```python
from build123d import *

# Parameters (mm, degrees)
SKETCH_1_W      = 100
SKETCH_1_H      = 70
EXTRUDE_1_DEPTH = 3.2


with BuildPart() as part:
    # Эскиз1 → Бобышка-Вытянуть1 (new body)
    with BuildSketch(Plane(origin=(0, 0, 0), x_dir=(1, 0, 0), z_dir=(0, 1, 0))):
        Rectangle(SKETCH_1_W, SKETCH_1_H)
        with BuildLine():
            Line((-42.453867058, 30.513030215), (-33.354611201, 5.513030215))
            ThreePointArc((-33.354611201, 5.513030215), (-34.251119917, 3.590461069), (-36.173689063, 4.486969785))
            Line((-36.173689063, 4.486969785), (-45.27294492, 29.486969785))
            ThreePointArc((-45.27294492, 29.486969785), (-44.376436204, 31.409538931), (-42.453867058, 30.513030215))
        make_face(mode=Mode.SUBTRACT)
        with BuildLine():
            Line((-32.453867058, 30.513030215), (-23.354611201, 5.513030215))
            ThreePointArc((-23.354611201, 5.513030215), (-24.251119917, 3.590461069), (-26.173689063, 4.486969785))
            Line((-26.173689063, 4.486969785), (-35.27294492, 29.486969785))
            ThreePointArc((-35.27294492, 29.486969785), (-34.376436204, 31.409538931), (-32.453867058, 30.513030215))
        make_face(mode=Mode.SUBTRACT)
        with BuildLine():
            Line((-22.453867058, 30.513030215), (-13.354611201, 5.513030215))
            ThreePointArc((-13.354611201, 5.513030215), (-14.251119917, 3.590461069), (-16.173689063, 4.486969785))
            Line((-16.173689063, 4.486969785), (-25.27294492, 29.486969785))
            ThreePointArc((-25.27294492, 29.486969785), (-24.376436204, 31.409538931), (-22.453867058, 30.513030215))
        make_face(mode=Mode.SUBTRACT)
        with BuildLine():
            Line((-12.453867058, 30.513030215), (-3.354611201, 5.513030215))
            ThreePointArc((-3.354611201, 5.513030215), (-4.251119917, 3.590461069), (-6.173689063, 4.486969785))
            Line((-6.173689063, 4.486969785), (-15.27294492, 29.486969785))
            ThreePointArc((-15.27294492, 29.486969785), (-14.376436204, 31.409538931), (-12.453867058, 30.513030215))
        make_face(mode=Mode.SUBTRACT)
        with BuildLine():
            Line((-2.453867058, 30.513030215), (6.645388799, 5.513030215))
            ThreePointArc((6.645388799, 5.513030215), (5.748880083, 3.590461069), (3.826310937, 4.486969785))
            Line((3.826310937, 4.486969785), (-5.27294492, 29.486969785))
            ThreePointArc((-5.27294492, 29.486969785), (-4.376436204, 31.409538931), (-2.453867058, 30.513030215))
        make_face(mode=Mode.SUBTRACT)
        with BuildLine():
            Line((7.546132942, 30.513030215), (16.645388799, 5.513030215))
            ThreePointArc((16.645388799, 5.513030215), (15.748880083, 3.590461069), (13.826310937, 4.486969785))
            Line((13.826310937, 4.486969785), (4.72705508, 29.486969785))
            ThreePointArc((4.72705508, 29.486969785), (5.623563796, 31.409538931), (7.546132942, 30.513030215))
        make_face(mode=Mode.SUBTRACT)
        with BuildLine():
            Line((17.546132942, 30.513030215), (26.645388799, 5.513030215))
            ThreePointArc((26.645388799, 5.513030215), (25.748880083, 3.590461069), (23.826310937, 4.486969785))
            Line((23.826310937, 4.486969785), (14.72705508, 29.486969785))
            ThreePointArc((14.72705508, 29.486969785), (15.623563796, 31.409538931), (17.546132942, 30.513030215))
        make_face(mode=Mode.SUBTRACT)
        with BuildLine():
            Line((27.546132942, 30.513030215), (36.645388799, 5.513030215))
            ThreePointArc((36.645388799, 5.513030215), (35.748880083, 3.590461069), (33.826310937, 4.486969785))
            Line((33.826310937, 4.486969785), (24.72705508, 29.486969785))
            ThreePointArc((24.72705508, 29.486969785), (25.623563796, 31.409538931), (27.546132942, 30.513030215))
        make_face(mode=Mode.SUBTRACT)
        with BuildLine():
            Line((37.546132942, 30.513030215), (46.645388799, 5.513030215))
            ThreePointArc((46.645388799, 5.513030215), (45.748880083, 3.590461069), (43.826310937, 4.486969785))
            Line((43.826310937, 4.486969785), (34.72705508, 29.486969785))
            ThreePointArc((34.72705508, 29.486969785), (35.623563796, 31.409538931), (37.546132942, 30.513030215))
        make_face(mode=Mode.SUBTRACT)
        with BuildLine():
            Line((-2.453867058, -30.513030215), (6.645388799, -5.513030215))
            ThreePointArc((6.645388799, -5.513030215), (5.748880083, -3.590461069), (3.826310937, -4.486969785))
            Line((3.826310937, -4.486969785), (-5.27294492, -29.486969785))
            ThreePointArc((-5.27294492, -29.486969785), (-4.376436204, -31.409538931), (-2.453867058, -30.513030215))
        make_face(mode=Mode.SUBTRACT)
        with BuildLine():
            Line((37.546132942, -30.513030215), (46.645388799, -5.513030215))
            ThreePointArc((46.645388799, -5.513030215), (45.748880083, -3.590461069), (43.826310937, -4.486969785))
            Line((43.826310937, -4.486969785), (34.72705508, -29.486969785))
            ThreePointArc((34.72705508, -29.486969785), (35.623563796, -31.409538931), (37.546132942, -30.513030215))
        make_face(mode=Mode.SUBTRACT)
        with BuildLine():
            Line((27.546132942, -30.513030215), (36.645388799, -5.513030215))
            ThreePointArc((36.645388799, -5.513030215), (35.748880083, -3.590461069), (33.826310937, -4.486969785))
            Line((33.826310937, -4.486969785), (24.72705508, -29.486969785))
            ThreePointArc((24.72705508, -29.486969785), (25.623563796, -31.409538931), (27.546132942, -30.513030215))
        make_face(mode=Mode.SUBTRACT)
        with BuildLine():
            Line((17.546132942, -30.513030215), (26.645388799, -5.513030215))
            ThreePointArc((26.645388799, -5.513030215), (25.748880083, -3.590461069), (23.826310937, -4.486969785))
            Line((23.826310937, -4.486969785), (14.72705508, -29.486969785))
            ThreePointArc((14.72705508, -29.486969785), (15.623563796, -31.409538931), (17.546132942, -30.513030215))
        make_face(mode=Mode.SUBTRACT)
        with BuildLine():
            Line((7.546132942, -30.513030215), (16.645388799, -5.513030215))
            ThreePointArc((16.645388799, -5.513030215), (15.748880083, -3.590461069), (13.826310937, -4.486969785))
            Line((13.826310937, -4.486969785), (4.72705508, -29.486969785))
            ThreePointArc((4.72705508, -29.486969785), (5.623563796, -31.409538931), (7.546132942, -30.513030215))
        make_face(mode=Mode.SUBTRACT)
        with BuildLine():
            Line((-12.453867058, -30.513030215), (-3.354611201, -5.513030215))
            ThreePointArc((-3.354611201, -5.513030215), (-4.251119917, -3.590461069), (-6.173689063, -4.486969785))
            Line((-6.173689063, -4.486969785), (-15.27294492, -29.486969785))
            ThreePointArc((-15.27294492, -29.486969785), (-14.376436204, -31.409538931), (-12.453867058, -30.513030215))
        make_face(mode=Mode.SUBTRACT)
        with BuildLine():
            Line((-22.453867058, -30.513030215), (-13.354611201, -5.513030215))
            ThreePointArc((-13.354611201, -5.513030215), (-14.251119917, -3.590461069), (-16.173689063, -4.486969785))
            Line((-16.173689063, -4.486969785), (-25.27294492, -29.486969785))
            ThreePointArc((-25.27294492, -29.486969785), (-24.376436204, -31.409538931), (-22.453867058, -30.513030215))
        make_face(mode=Mode.SUBTRACT)
        with BuildLine():
            Line((-32.453867058, -30.513030215), (-23.354611201, -5.513030215))
            ThreePointArc((-23.354611201, -5.513030215), (-24.251119917, -3.590461069), (-26.173689063, -4.486969785))
            Line((-26.173689063, -4.486969785), (-35.27294492, -29.486969785))
            ThreePointArc((-35.27294492, -29.486969785), (-34.376436204, -31.409538931), (-32.453867058, -30.513030215))
        make_face(mode=Mode.SUBTRACT)
        with BuildLine():
            Line((-42.453867058, -30.513030215), (-33.354611201, -5.513030215))
            ThreePointArc((-33.354611201, -5.513030215), (-34.251119917, -3.590461069), (-36.173689063, -4.486969785))
            Line((-36.173689063, -4.486969785), (-45.27294492, -29.486969785))
            ThreePointArc((-45.27294492, -29.486969785), (-44.376436204, -31.409538931), (-42.453867058, -30.513030215))
        make_face(mode=Mode.SUBTRACT)
    extrude(amount=EXTRUDE_1_DEPTH)


solid = part.part
```
Input: part model. Units: mm. Frame: model coordinates. Coordinates: 2 decimals unless noted, no trailing zeros. Loops run counter-clockwise (first coordinate to the right, second up) from the corner with the lowest first, then second, coordinate; pieces in that order, holes last. Notation, with made-up numbers: M 65.25,79 L 90.25,79 A25 ccw 90.25,117 Z; hole C -1,-30.75 d10. An arc over 180 degrees is marked long. Use a Markdown table: item, result. Add a question column.
1) Section A-A, the plane x = -28.5. Return the cut outline in (y, z), plus the area to 3 significant figures.
2) Section B-B, the plane y = 2.05. Give the number of separate pieces and of enclosed holes in the cut face, plus the area to 3 significant figures.
3) Draft query along X for faces 1 (the flat face through (-1, 2, 35)), 2 (the cylindrical face through (-24.4, 1.6, -31.4)), 3 (the flat face through (-20.66, 1.58, 16.81)), 4 (the flat face through (50, 2, 0)). Return one class per face: +X half, -X half, draft (parallel to the pull), parting line (faces both ways), or undercut.
4) Pin query (flat end, axial travel): P1, Ø5, axis at x = -34.5, z = 3, coming from the -Y side. Return the tip coordinate at first contact, or that it passes through.
Answer below:
| question | item | result |
|---|---|---|
| 1 | outline | M 0,-35 L 3.2,-35 L 3.2,-19.65 L 0,-19.65 Z; M 0,-10.88 L 3.2,-10.88 L 3.2,10.88 L 0,10.88 Z; M 0,19.65 L 3.2,19.65 L 3.2,35 L 0,35 Z |
| 1 | area | 168 mm2 |
| 2 | separate pieces | 1 |
| 2 | enclosed holes | 18 |
| 2 | area | 5,440 mm2 |
| 3 | face 1 | draft |
| 3 | face 2 | undercut |
| 3 | face 3 | undercut |
| 3 | face 4 | +X half |
| 4 | P1 | y = 0 |
